Verification items for the finished model (mm, model axes). A direction names the side the tool comes from. Give positions to 0.01 mm unless a question says otherwise; leave off trailing zeros. Write each loop counter-clockwise with the first axis right and the second up, starting at its lowest first coordinate (ties: lowest second). Pieces come first, ordered by that corner, then holes. Notation, with made-up numbers: (-32.5, -32) -> (-12.5, -32) arc R25 cw to (-12.5, -13) -> close; hole circle Ø8 at (76, -38.75). An arc over 180 degrees is marked (long way). Answer as CSV lines item,"result". Start each with the question number.
1) Sectioned sample at A-A on x = 20.3. Record the cut outline in (y, z), and give its area (3 significant figures).
2) Material ranges on L1, parallel to Y at x = 1, z = -6.8; L2, parallel to X at y = 50.5, z = -21.75; L3, parallel to Y at x = 1.2, z = -6.8, recorded low to high.
3) Sectioned sample at B-B on x = 27.5. Record the cut outline in (y, z).
4) Tool access check on faces 5 (the cylindrical face through (53.8, 11.5, -23.5)), 6 (the flat face through (2.5, 35, -14)), 7 (the cylindrical face through (1.3, 58.3, -4)). Record the directions out of +Z, -Z, +X, -X, +Y, -Y that give a thin tool (end or side, any length) a straight path to the whole face; none if there is none.
5) Gauge pin test, flat ends, axial feed: pin 1 Ø1.5 at (x, z) = (22.5, -23.5) entering from +Y; pin 2 Ø2 at (y, z) = (53.59, -19.09) entering from +X; pin 3 Ø0.8 at (x, z) = (53.5, -13) entering from +Y; pin 4 Ø5 at (x, z) = (9, -5.5) entering from +Y. Record the tip position at first contact, or that the pin passes through.
6) Mould release check, pull along X, two halves, no side actions. Record for faces 1 (the cylindrical face through (31.704, 1.232, -18.63)), 2 (the flat face through (0, 39, -14)), 3 (the flat face through (54, 34, -14)), 4 (the cylindrical face through (21.52, 1.23, -8.45)): released by +X, released by -X, zero draft, split by the parting line, or undercut.
7) Sectioned sample at D-D on y = 41.3. Record the cut outline in (x, z), and give its area (3 significant figures).
8) Sectioned sample at C-C on y = 30. Record the cut outline in (x, z), and give its area (3 significant figures).
```python
from build123d import *

# Parameters (mm, degrees)
ESQUISSE1_W             = 55
ESQUISSE1_H             = 28
ESQUISSE1_R             = 1
ESQUISSE1_R_2           = 3
BOSS_EXTRU_1_DEPTH      = 2.5
ESQUISSE2_W             = 2.5
ESQUISSE2_H             = 28
BOSS_EXTRU_2_DEPTH      = 60
CONG_1_R                = 5
CONG_2_R                = 2
ESQUISSE3_R             = 1.224893227
ESQUISSE3_R_2           = 3
ENL_V_MAT_EXTRU_1_DEPTH = 55
CONG_3_R                = 14


with BuildPart() as part:
    # Esquisse1 → Boss.-Extru.1 (new body)
    with BuildSketch(Plane(origin=(0, 0, 0), x_dir=(1, 0, 0), z_dir=(0, 1, 0))):
        with Locations((27.5, 14)):
            Rectangle(ESQUISSE1_W, ESQUISSE1_H)
        with Locations(Location((22.408831175, 19.091168825, 0), (0, 0, 270))):
            Circle(ESQUISSE1_R, mode=Mode.SUBTRACT)
        with Locations(Location((27.5, 21.2, 0), (0, 0, 270))):
            Circle(ESQUISSE1_R, mode=Mode.SUBTRACT)
        with Locations(Location((32.591168825, 19.091168825, 0), (0, 0, 270))):
            Circle(ESQUISSE1_R, mode=Mode.SUBTRACT)
        with Locations(Location((34.7, 14, 0), (0, 0, 270))):
            Circle(ESQUISSE1_R, mode=Mode.SUBTRACT)
        with Locations(Location((32.591168825, 8.908831175, 0), (0, 0, 270))):
            Circle(ESQUISSE1_R, mode=Mode.SUBTRACT)
        with Locations(Location((27.5, 6.8, 0), (0, 0, 270))):
            Circle(ESQUISSE1_R, mode=Mode.SUBTRACT)
        with Locations(Location((22.408831175, 8.908831175, 0), (0, 0, 270))):
            Circle(ESQUISSE1_R, mode=Mode.SUBTRACT)
        with Locations(Location((20.3, 14, 0), (0, 0, 270))):
            Circle(ESQUISSE1_R, mode=Mode.SUBTRACT)
        with Locations(Location((27.5, 14, 0), (0, 0, 270))):
            Circle(ESQUISSE1_R_2, mode=Mode.SUBTRACT)
    extrude(amount=BOSS_EXTRU_1_DEPTH)

    # Esquisse2 → Boss.-Extru.2 (add)
    with BuildSketch(Plane(origin=(0, 2.5, 0), x_dir=(1, 0, 0), z_dir=(0, 1, 0))):
        with Locations((1.25, 14)):
            Rectangle(ESQUISSE2_W, ESQUISSE2_H)
        with Locations((53.75, 14)):
            Rectangle(ESQUISSE2_W, ESQUISSE2_H)
    extrude(amount=BOSS_EXTRU_2_DEPTH)

    # Congé1
    cong_1_edges = [part.edges().sort_by_distance(p)[0] for p in [
        (2.5, 2.5, -14),
        (52.5, 2.5, -14),
    ]]
    fillet(cong_1_edges, radius=CONG_1_R)

    # Congé2
    cong_2_edges = [part.edges().sort_by_distance(p)[0] for p in [
        (55, 0, -14),
        (0, 0, -14),
    ]]
    fillet(cong_2_edges, radius=CONG_2_R)

    # Esquisse3 → Enlèv. mat.-Extru.1 (cut)
    with BuildSketch(Plane(origin=(55, 0, 0), x_dir=(0, 0, -1), z_dir=(1, 0, 0))):
        with Locations((14, 41.3)):
            Circle(ESQUISSE3_R)
        with Locations((8.908831175, 43.408831175)):
            Circle(ESQUISSE3_R)
        with Locations((6.8, 48.5)):
            Circle(ESQUISSE3_R)
        with Locations((8.908831175, 53.591168825)):
            Circle(ESQUISSE3_R)
        with Locations((14, 55.7)):
            Circle(ESQUISSE3_R)
        with Locations((19.091168825, 53.591168825)):
            Circle(ESQUISSE3_R)
        with Locations((21.2, 48.5)):
            Circle(ESQUISSE3_R)
        with Locations((19.091168825, 43.408831175)):
            Circle(ESQUISSE3_R)
        with Locations((14, 48.5)):
            Circle(ESQUISSE3_R_2)
        with BuildLine():
            Line((22, 10), (6, 10))
            ThreePointArc((6, 10), (4.5, 11.5), (6, 13))
            Line((6, 13), (22, 13))
            ThreePointArc((22, 13), (23.5, 11.5), (22, 10))
        make_face()
        with BuildLine():
            Line((22, 17), (6, 17))
            ThreePointArc((6, 17), (4.5, 18.5), (6, 20))
            Line((6, 20), (22, 20))
            ThreePointArc((22, 20), (23.5, 18.5), (22, 17))
        make_face()
        with BuildLine():
            Line((22, 24), (6, 24))
            ThreePointArc((6, 24), (4.5, 25.5), (6, 27))
            Line((6, 27), (22, 27))
            ThreePointArc((22, 27), (23.5, 25.5), (22, 24))
        make_face()
        with BuildLine():
            Line((22, 31), (6, 31))
            ThreePointArc((6, 31), (4.5, 32.5), (6, 34))
            Line((6, 34), (22, 34))
            ThreePointArc((22, 34), (23.5, 32.5), (22, 31))
        make_face()
    extrude(amount=-ENL_V_MAT_EXTRU_1_DEPTH, mode=Mode.SUBTRACT)

    # Congé3
    cong_3_edges = [part.edges().sort_by_distance(p)[0] for p in [
        (1.25, 62.5, 0),
        (53.75, 62.5, -28),
        (53.75, 62.5, 0),
        (1.25, 62.5, -28),
    ]]
    fillet(cong_3_edges, radius=CONG_3_R - 0.0001)  # a hair under: the kernel refuses the full size


solid = part.part
```
Ans:
1,outline,"(0, -28) -> (2.5, -28) -> (2.5, -15) -> (0, -15) -> close; (0, -13) -> (2.5, -13) -> (2.5, 0) -> (0, 0) -> close"
1,area,"65.0 mm²"
2,L1,"y = 0.27 to 10, 13 to 17, 20 to 24, 27 to 31, 34 to 47.28, 49.72 to 60.51"
2,L2,"x = 0 to 2.5, 52.5 to 55"
2,L3,"y = 0.17 to 10, 13 to 17, 20 to 24, 27 to 31, 34 to 47.28, 49.72 to 60.51"
3,outline,"(0, -28) -> (2.5, -28) -> (2.5, -22.2) -> (0, -22.2) -> close; (0, -20.2) -> (2.5, -20.2) -> (2.5, -17) -> (0, -17) -> close; (0, -11) -> (2.5, -11) -> (2.5, -7.8) -> (0, -7.8) -> close; (0, -5.8) -> (2.5, -5.8) -> (2.5, 0) -> (0, 0) -> close"
4,face 5,"+X, -X"
4,face 6,"+Z, -Z, +Y"
4,face 7,"+Z, +X, -X, +Y"
5,pin 1,"stops at y = 2.5"
5,pin 2,"passes through"
5,pin 3,"stops at y = 62.49"
5,pin 4,"stops at y = 2.6"
6,face 1,"undercut"
6,face 2,"released by -X"
6,face 3,"zero draft"
6,face 4,"undercut"
7,outline,"(0, -28) -> (2.5, -28) -> (2.5, -15.22) -> (0, -15.22) -> close; (0, -12.78) -> (2.5, -12.78) -> (2.5, 0) -> (0, 0) -> close; (52.5, -28) -> (55, -28) -> (55, -15.22) -> (52.5, -15.22) -> close; (52.5, -12.78) -> (55, -12.78) -> (55, 0) -> (52.5, 0) -> close"
7,area,"128 mm²"
8,outline,"(0, -28) -> (2.5, -28) -> (2.5, 0) -> (0, 0) -> close; (52.5, -28) -> (55, -28) -> (55, 0) -> (52.5, 0) -> close"
8,area,"140 mm²"
